Can you work these out from the drawing? Everything is in mm from the part's minimum corner. Round coordinates to 2 decimals unless told otherwise and drop trailing zeros. Loops run counter-clockwise (first coordinate to the right, second up) from the corner with the lowest first, then second, coordinate; pieces in that order, holes last. Notation, with made-up numbers: (13, -24) -> (52, -24) arc R23 cw to (52, -8) -> close; hole circle Ø1 at (39.25, -17.75). An arc over 180 degrees is marked (long way). One line per item, written item: value.
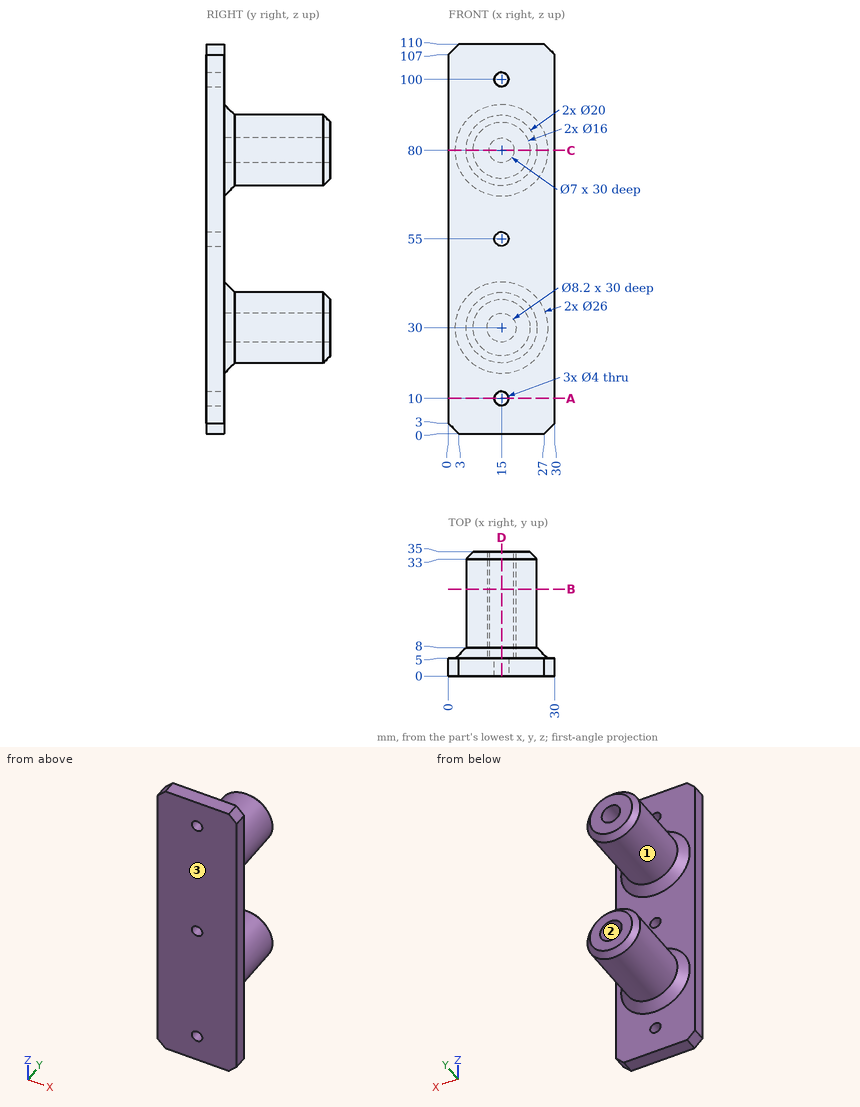
Item 1: If we section it at B-B on y = 24.5: List the corners of the cut face in (x, z) for me.
Output:
outline: circle Ø20 at (15, 30); circle Ø20 at (15, 80); hole circle Ø8.2 at (15, 30); hole circle Ø7 at (15, 80)
Item 2: I need wall thicknesses on line 1 (Z direction, x = 15, y = 3.35); line 2 (Z direction, x = 15, y = 23.75); line 3 (X direction, y = 3.3, z = 55). Which ranges of each line are inside material? Lowest first, please. Write a range as from..to.
Output:
line 1: z = 0..8, 12..53, 57..98, 102..110
line 2: z = 20..25.9, 34.1..40, 70..76.5, 83.5..90
line 3: x = 0..13, 17..30
Item 3: If we section it at C-C on z = 80: List the corners of the cut face in (x, y) for me.
Output:
outline: (0, 0) -> (30, 0) -> (30, 5) -> (28, 5) -> (25, 8) -> (25, 33) -> (23, 35) -> (18.5, 35) -> (18.5, 5) -> (11.5, 5) -> (11.5, 35) -> (7, 35) -> (5, 33) -> (5, 8) -> (2, 5) -> (0, 5) -> close
Item 4: If we section it at D-D on x = 15: Count the separate pieces of the cut face and the enclosed holes in it, plus the area to 3 significant figures.
Output:
separate pieces: 4
enclosed holes: 0
area: 1,240 mm²
Item 5: If we mould it in two halves opening along X, with no side actions, what happens to the marked faces 1, 2 and 3? For each: released by +X, released by -X, zero draft, split by the parting line, or undercut.
Output:
face 1: split by the parting line
face 2: undercut
face 3: zero draft
Item 6: If we section it at A-A on z = 10: List the corners of the cut face in (x, y) for me.
Output:
outline: (0, 0) -> (13, 0) -> (13, 5) -> (0, 5) -> close; (17, 0) -> (30, 0) -> (30, 5) -> (17, 5) -> close
Item 7: Will these pins go through, and if not, where does the flat tip stop? pin 1 Ø3.5 at (x, z) = (16.5, 80.5) entering from +Y; pin 2 Ø10 at (y, z) = (21.5, 32) entering from +X; pin 3 Ø6 at (y, z) = (23.5, 15.5) entering from +X; pin 4 Ø4 at (x, y) = (24, 21.5) entering from +Z.
Output:
pin 1: stops at y = 5
pin 2: stops at x = 25
pin 3: passes through
pin 4: stops at z = 87.14
